Source: CAD feature listing. Evaluate the final solid. Frame: model axes, mm. A direction names the side the tool comes from. Coordinates: 2 decimals unless noted, no trailing zeros. Order: outer loops, then holes, each group sorted by start corner. A loop starts at its lowest first (then second) coordinate and runs counter-clockwise, first axis right, second up. Notation, with made-up numbers: (61.5, 85) -> (72.5, 85) arc R17 ccw to (72.5, 94) -> close; hole circle Ø5 at (8, 9). An arc over 180 degrees is marked (long way). Put each result on its own line as item: value.
from build123d import *

# Parameters (mm, degrees)
SKETCH1_R           = 11
BOSS_EXTRUDE1_DEPTH = 2
SKETCH2_R           = 5
BOSS_EXTRUDE2_DEPTH = 10
SKETCH3_R           = 2
CUT_EXTRUDE1_DEPTH  = 13
CHAMFER1_SIZE       = 0.5
SKETCH4_R           = 1.5
CUT_EXTRUDE2_DEPTH  = 10


with BuildPart() as part:
    # Sketch1 → Boss-Extrude1 (new body)
    with BuildSketch(Plane(origin=(0, 0, 0), x_dir=(1, 0, 0), z_dir=(0, 1, 0))):
        Circle(SKETCH1_R)
    extrude(amount=BOSS_EXTRUDE1_DEPTH)

    # Sketch2 → Boss-Extrude2 (add)
    with BuildSketch(Plane(origin=(0, 2, 0), x_dir=(1, 0, 0), z_dir=(0, 1, 0))):
        Circle(SKETCH2_R)
    extrude(amount=BOSS_EXTRUDE2_DEPTH)

    # Sketch3 → Cut-Extrude1 (cut, through all)
    with BuildSketch(Plane(origin=(0, 12, 0), x_dir=(1, 0, 0), z_dir=(0, 1, 0))):
        Circle(SKETCH3_R)
    extrude(amount=-CUT_EXTRUDE1_DEPTH, mode=Mode.SUBTRACT)

    # Chamfer1
    chamfer1_edges = [part.edges().sort_by_distance(p)[0] for p in [
        (-5, 12, 0),
    ]]
    chamfer(chamfer1_edges, length=CHAMFER1_SIZE)

    # Sketch4 → Cut-Extrude2 (cut)
    with BuildSketch(Plane.XZ):
        with Locations((-5.656854249, 5.656854249)):
            Circle(SKETCH4_R)
        with Locations((5.656854249, 5.656854249)):
            Circle(SKETCH4_R)
        with Locations((5.656854249, -5.656854249)):
            Circle(SKETCH4_R)
        with Locations((-5.656854249, -5.656854249)):
            Circle(SKETCH4_R)
    extrude(amount=-CUT_EXTRUDE2_DEPTH, mode=Mode.SUBTRACT)


solid = part.part
1. Ray query, line 1 along X through (y, z) = (7.5, 0); line 2 along Y through (x, z) = (6, 4); line 3 along X through (y, z) = (4.5, 1.75). Return the intervals inside material, ascending.
Numbers:
line 1: x = -5 to -2, 2 to 5
line 2: y = 0 to 2
line 3: x = -4.68 to -0.97, 0.97 to 4.68
2. Set-up query: faces 1 (the flat face through (2, 2, 5)), 2 (the flat face through (-0.2, 0, 2.3)). Return all of +Z, -Z, +X, -X, +Y, -Y with unobstructed straight access to the full face (end or side cutting, diameter ignored); none if empty.
Numbers:
face 1: +Y
face 2: +Z, -Z, +X, -X, -Y
3. Cut plane C-C on y = 3.25. Output: boundary loops of the cut face in (x, z).
Numbers:
outline: circle Ø10 at (0, 0); hole circle Ø4 at (0, 0)
4. Cut plane D-D on x = 7.5. Output: boundary loops of the cut face in (y, z), plus the area to 3 significant figures.
Numbers:
outline: (0, -8.05) -> (2, -8.05) -> (2, 8.05) -> (0, 8.05) -> close
area: 32.2 mm2
5. Cut plane B-B on z = 0. Output: boundary loops of the cut face in (x, y), plus the area to 4 significant figures.
Numbers:
outline: (-11, 0) -> (-2, 0) -> (-2, 12) -> (-4.5, 12) -> (-5, 11.5) -> (-5, 2) -> (-11, 2) -> close; (2, 0) -> (11, 0) -> (11, 2) -> (5, 2) -> (5, 11.5) -> (4.5, 12) -> (2, 12) -> close
area: 95.75 mm2
6. Pull-direction query (X, two-part tool) for faces 3 (the cylindrical face through (6.3, 1, 4.3)), 4 (the cylindrical face through (-1.08, 6.68, 4.88)), 5 (the cylindrical face through (-5.85, 0.99, -4.17)), 6 (the flat face through (1, 12, 2)); classes: pulls with the +X half, pulls with the -X half, needs draft (parallel to the pull), parting line crosses it, or undercut.
Numbers:
face 3: undercut
face 4: parting line crosses it
face 5: undercut
face 6: needs draft
7. First-contact query: pin 1 (1.5 mm diameter, centred on x = 4.5, y = 6.5, fed in from -Z); pin 2 (5 mm diameter, centred on x = 3.5, y = 6, fed in from -Z); pin 3 (4 mm diameter, centred on y = 10, z = 4.5, fed in from -X). Flat tips, straight axial feed; report the tip coordinate or a pass-through.
Numbers:
pin 1: stops at z = -3.31
pin 2: stops at z = -4.9
pin 3: stops at x = -4.33
8. Cut plane A-A on x = 0. Output: boundary loops of the cut face in (y, z).
Numbers:
outline: (0, -11) -> (2, -11) -> (2, -5) -> (11.5, -5) -> (12, -4.5) -> (12, -2) -> (0, -2) -> close; (0, 2) -> (12, 2) -> (12, 4.5) -> (11.5, 5) -> (2, 5) -> (2, 11) -> (0, 11) -> close
